Read the model definition and answer for the solid it produces. Units are mm, in the model's axes. Face numbers are marked on the shaded views. A direction names the side the tool comes from. Coordinates: 2 decimals unless noted, no trailing zeros. Order: outer loops, then holes, each group sorted by start corner. A loop starts at its lowest first (then second) coordinate and runs counter-clockwise, first axis right, second up.
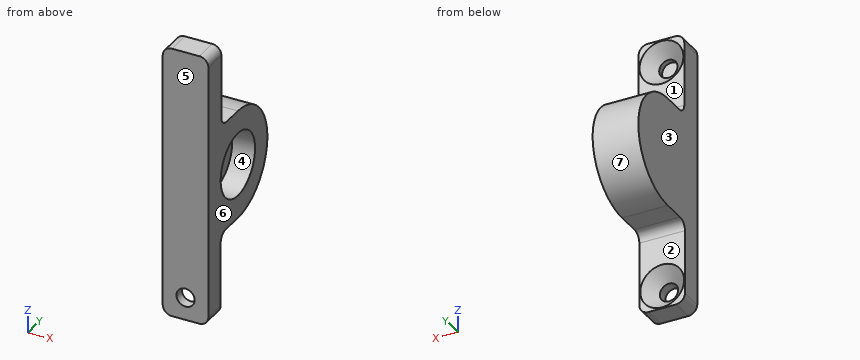
Autodesk Inventor part; units mm, degrees
ref_plane "YZ Plane" through (0, 0, 0) normal (1, 0, 0) x (0, 1, 0)
ref_plane "XZ Plane" through (0, 0, 0) normal (0, 1, 0) x (-1, 0, 0)
ref_plane "XY Plane" through (0, 0, 0) normal (0, 0, 1) x (1, 0, 0)
sketch "Sketch1" plane through (0, 0, 0) normal (1, 0, 0) x (0, 1, 0)
  circle A0 centre (0, 0) radius 7
  arc A1 (0, -12) -> (0, 12) centre (0, 0) ccw
  circle A2 centre (0, 0) radius 2.475
  line L0 (-12, -30) -> (-12, 29.9986)
  line L1 (-6.7144, 29.9986) -> (-12, 29.9986)
  line L2 (-12, -30) -> (-7, -30)
  line L3 (-7, -30) -> (-7, -12)
  line L4 (0, -12) -> (-7, -12)
  line L5 (0, 12) -> (-6.7144, 12)
  line L6 (-6.7144, 12) -> (-6.7144, 29.9986)
  point P0 (-7, 0)
  dimension "d0" = 14
  dimension "d1" = 30
  dimension "d2" = 30
  dimension "d4" = 5
  dimension "d5" = 4.95
  dimension "d22" = 5
extrude "Extrusion1" add sketch "Sketch1" along normal blind 5 contours A0 | A2
extrude "Extrusion2" add sketch "Sketch1" along normal blind 10 contours L4 L3 L2 L0 L1 L6 L5 A1
sketch "Sketch3" plane through (0, -7, -12) normal (0, 1, 0) x (1, 0, 0)
  circle A0 centre (5, 13) radius 2
  line L0 (0, 18) -> (10, 18)
  point P0 (0, -12)
  point P1 (5, 18)
  dimension "d26" = 4
  dimension "d27" = 0
  dimension "d28" = 5
extrude "Extrusion4" cut sketch "Sketch3" against normal blind 10
chamfer "Chamfer4" distance 2.8 angle 45 1 edges at (3, -7, -25)
fillet "Fillet2" radius 2 2 edges at (10, -9.5, -30) (0, -9.5, -30)
sketch "Sketch4" plane through (0, -6.7144, 29.9986) normal (0, 1, 0) x (1, 0, 0)
  circle A0 centre (5, 5) radius 2
  line L0 (0, 0) -> (10, 0)
  point P0 (0, 29.9986)
  point P1 (5, 0)
  dimension "d35" = 4
  dimension "d36" = 0
  dimension "d37" = 5
extrude "Extrusion5" cut sketch "Sketch4" against normal blind 4
chamfer "Chamfer5" distance 2.8 angle 45 1 edges at (3, -6.7144, 24.9986)
fillet "Fillet3" radius 2 4 edges at (0, -9.3572, 29.9986) (10, -9.3572, 29.9986) (5, -6.7144, 12) (5, -7, -12)
equation "\"d38\" = d35"
properties part number "bearing_holder"
1) A cutting plane is placed at A-A, the plane z = -25. Determine the outline of the cut face in (x, y).
A:
outline: (0, -12) - (3, -12) - (3, -9.8) - (0.2, -7) - (0, -7) - close; (7, -12) - (10, -12) - (10, -7) - (9.8, -7) - (7, -9.8) - close
2) Determine the mould class of the marked faces 4, 5, 6 and 7 for opening direction Y: pulls with the +Y half, pulls with the -Y half, needs draft (parallel to the pull), parting line crosses it, or undercut.
A:
face 4: undercut
face 5: pulls with the -Y half
face 6: needs draft
face 7: pulls with the +Y half
3) Which of the six approach directions +Z, -Z, +X, -X, +Y, -Y give full straight-line access (tool end or side, diameter ignored) to the marked faces 1, 2 and 3?
A:
face 1: +Z, +X, -X, +Y
face 2: -Z, +X, -X, +Y
face 3: +Z, -Z, -X, +Y, -Y
4) A cutting plane is placed at C-C, the plane y = 2. Determine the outline of the cut face in (x, z), and give its area (3 significant figures).
A:
outline: (0, -11.83) - (10, -11.83) - (10, -6.71) - (5, -6.71) - (5, 6.71) - (10, 6.71) - (10, 11.83) - (0, 11.83) - close
area: 170 mm2
5) Flat-ended cylindrical pins translate along their axes: pin 1 Ø4 at (y, z) = (-0.5, 1) entering from +X; pin 2 Ø3 at (x, z) = (5, -25) entering from +Y; pin 3 Ø1.5 at (x, y) = (7.5, 9) entering from -Z; pin 4 Ø3 at (x, y) = (5, 7.5) entering from -Z. Find the tip coordinate at first contact, or state that the pin passes through.
A:
pin 1: stops at x = 5
pin 2: passes through
pin 3: stops at z = -8.71
pin 4: stops at z = -10.39
6) A cutting plane is placed at D-D, the plane z = 19.5. Determine the outline of the cut face in (x, y).
A:
outline: (0, -12) - (10, -12) - (10, -6.71) - (0, -6.71) - close
7) A cutting plane is placed at B-B, the plane z = 0. Determine the outline of the cut face in (x, y).
A:
outline: (0, -12) - (10, -12) - (10, -7) - (5, -7) - (5, 7) - (10, 7) - (10, 12) - (0, 12) - close
8) Straight lines are drawn through the part: line 1 (Z direction, x = 5, y = -9.85); line 2 (Z direction, x = 7.65, y = 0); line 3 (X direction, y = -10.75, z = -25). For each, find the intervals that lie inside material, in ascending order.
A:
line 1: z = -30 to -27, -23 to 23, 27 to 30
line 2: z = -12 to -7, 7 to 12
line 3: x = 0 to 3, 7 to 10
